Could you check a few things on this model? Use its own coordinates, in mm. A direction names the side the tool comes from. Give positions to 0.01 mm unless a question says otherwise; leave off trailing zeros. Loops run counter-clockwise (first coordinate to the right, second up) from the corner with the lowest first, then second, coordinate; pieces in that order, holes last. Notation, with made-up numbers: (32.25, 40) -> (56.25, 40) arc R17 ccw to (56.25, 52) -> close; hole circle Ø2 at (-39.5, 82.5). An arc over 180 degrees is marked (long way). Write item = value, one per line. Start each with the question number.
1) On a 3-axis mill with a long thin cutter (end or side, diameter ignored), from which of +Z, -Z, +X, -X, +Y, -Y can I reach the whole of each face in a straight line? I mean faces 1 (the face through (-7.094, 44.219, 1.479)), 2 (the face through (49, -0.5, 1)), 3 (the face through (50, 46.5, 1)). Say none if no direction works.
2) If we mould it in two halves opening along Y, with no side actions, what happens to faces 4 (the face through (58.219, 44.094, 1.479)), 5 (the face through (13, 31.57, 1.52)), 6 (the face through (25, 23, 3))? For each: +Y half, -Y half, draft (parallel to the pull), parting line (faces both ways), or undercut.
3) I need wall thicknesses on probe 1 along Y at (x, z) = (14.5, 0.7); probe 2 along Y at (x, z) = (32.5, 0.6); probe 3 along Y at (x, z) = (-1.5, 1.5). Which ranges of each line are inside material? Lowest first, please. Write a range as from..to.
4) I want a section at D-D (y = 1). List the corners of the cut face in (x, z) for me, and give its area (3 significant figures).
5) I want a section at A-A (z = 0.95). List the corners of the cut face in (x, y) for me.
6) I'm going to push flat-ended pins straight in: pin 1 Ø0.8 at (y, z) = (-1, 1.5) entering from +X; pin 2 Ø1 at (x, z) = (44, 2) entering from +Y (3 decimals); pin 3 Ø1 at (y, z) = (2, 2) entering from +X (3 decimals). Where does each tip first touch, or does it pass through?
7) I want a section at B-B (y = 14.5). List the corners of the cut face in (x, z) for me.
8) I want a section at C-C (x = 31.5). List the corners of the cut face in (y, z) for me.
from build123d import *

# Parameters (mm, degrees)
RESSALTO_EXTRUS_O1_DEPTH = 3
ESBO_O5_R                = 1.5
CORTE_EXTRUS_O1_DEPTH    = 4


with BuildPart() as part:
    # Esboço1 → Ressalto-extrusão1 (new body)
    with BuildSketch(Plane.XY):
        with BuildLine():
            Line((7.5, -9.5), (38.5, -9.5))
            ThreePointArc((38.5, -9.5), (44.156854249, -7.156854249), (46.5, -1.5))
            Line((46.5, -1.5), (46.5, -0.5))
            Line((46.5, -0.5), (52.5, -0.5))
            ThreePointArc((52.5, -0.5), (58.156854249, 1.843145751), (60.5, 7.5))
            Line((60.5, 7.5), (60.5, 38.5))
            ThreePointArc((60.5, 38.5), (58.156854249, 44.156854249), (52.5, 46.5))
            Line((52.5, 46.5), (46.5, 46.5))
            Line((46.5, 46.5), (46.5, 47.5))
            ThreePointArc((46.5, 47.5), (44.156854249, 53.156854249), (38.5, 55.5))
            Line((38.5, 55.5), (7.5, 55.5))
            ThreePointArc((7.5, 55.5), (1.843145751, 53.156854249), (-0.5, 47.5))
            Line((-0.5, 47.5), (-0.5, 46.5))
            Line((-0.5, 46.5), (-1.5, 46.5))
            ThreePointArc((-1.5, 46.5), (-7.156854249, 44.156854249), (-9.5, 38.5))
            Line((-9.5, 38.5), (-9.5, 7.5))
            ThreePointArc((-9.5, 7.5), (-7.156854249, 1.843145751), (-1.5, -0.5))
            Line((-1.5, -0.5), (-0.5, -0.5))
            Line((-0.5, -0.5), (-0.5, -1.5))
            ThreePointArc((-0.5, -1.5), (1.843145751, -7.156854249), (7.5, -9.5))
        make_face()
    extrude(amount=RESSALTO_EXTRUS_O1_DEPTH)

    # Esboço5 → Corte-extrusão1 (cut, through all)
    with BuildSketch(Plane.XY.offset(3)):
        with Locations((31.5, 31.5)):
            Circle(ESBO_O5_R)
        with Locations((14.5, 31.5)):
            Circle(ESBO_O5_R)
        with Locations((14.5, 14.5)):
            Circle(ESBO_O5_R)
        with Locations((31.5, 14.5)):
            Circle(ESBO_O5_R)
    extrude(amount=-CORTE_EXTRUS_O1_DEPTH, mode=Mode.SUBTRACT)


solid = part.part
Answer list:
q1.face_1 = +Z, -Z, -X, +Y
q1.face_2 = +Z, -Z, +X, -Y
q1.face_3 = +Z, -Z, +X, +Y
q2.face_4 = +Y half
q2.face_5 = undercut
q2.face_6 = draft
q3.probe_1 = -9.5..13, 16..30, 33..55.5
q3.probe_2 = -9.5..13.38, 15.62..30.38, 32.62..55.5
q3.probe_3 = -0.5..46.5
q4.outline = (-6.16, 0) -> (57.16, 0) -> (57.16, 3) -> (-6.16, 3) -> close
q4.area = 190 mm^2
q5.outline = (-9.5, 7.5) arc R8 ccw to (-1.5, -0.5) -> (-0.5, -0.5) -> (-0.5, -1.5) arc R8 ccw to (7.5, -9.5) -> (38.5, -9.5) arc R8 ccw to (46.5, -1.5) -> (46.5, -0.5) -> (52.5, -0.5) arc R8 ccw to (60.5, 7.5) -> (60.5, 38.5) arc R8 ccw to (52.5, 46.5) -> (46.5, 46.5) -> (46.5, 47.5) arc R8 ccw to (38.5, 55.5) -> (7.5, 55.5) arc R8 ccw to (-0.5, 47.5) -> (-0.5, 46.5) -> (-1.5, 46.5) arc R8 ccw to (-9.5, 38.5) -> close; hole circle Ø3 at (14.5, 14.5); hole circle Ø3 at (14.5, 31.5); hole circle Ø3 at (31.5, 14.5); hole circle Ø3 at (31.5, 31.5)
q6.pin_1 = 46.5
q6.pin_2 = 53.745
q6.pin_3 = 58.745
q7.outline = (-9.5, 0) -> (13, 0) -> (13, 3) -> (-9.5, 3) -> close; (16, 0) -> (30, 0) -> (30, 3) -> (16, 3) -> close; (33, 0) -> (60.5, 0) -> (60.5, 3) -> (33, 3) -> close
q8.outline = (-9.5, 0) -> (13, 0) -> (13, 3) -> (-9.5, 3) -> close; (16, 0) -> (30, 0) -> (30, 3) -> (16, 3) -> close; (33, 0) -> (55.5, 0) -> (55.5, 3) -> (33, 3) -> close
